Verification items for this drawing (mm, ordinates from the low corner). Round coordinates to 2 decimals unless told otherwise and drop trailing zeros. Write each loop counter-clockwise with the first axis right and the second up, starting at its lowest first coordinate (ties: lowest second). Pieces come first, ordered by that corner, then holes. Notation, with made-up numbers: (-36.75, 31) -> (2.25, 31) arc R28 ccw to (2.25, 61) -> close; hole circle Ø4 at (59.25, -31.75). An arc over 180 degrees is marked (long way). One line per item, written item: value.
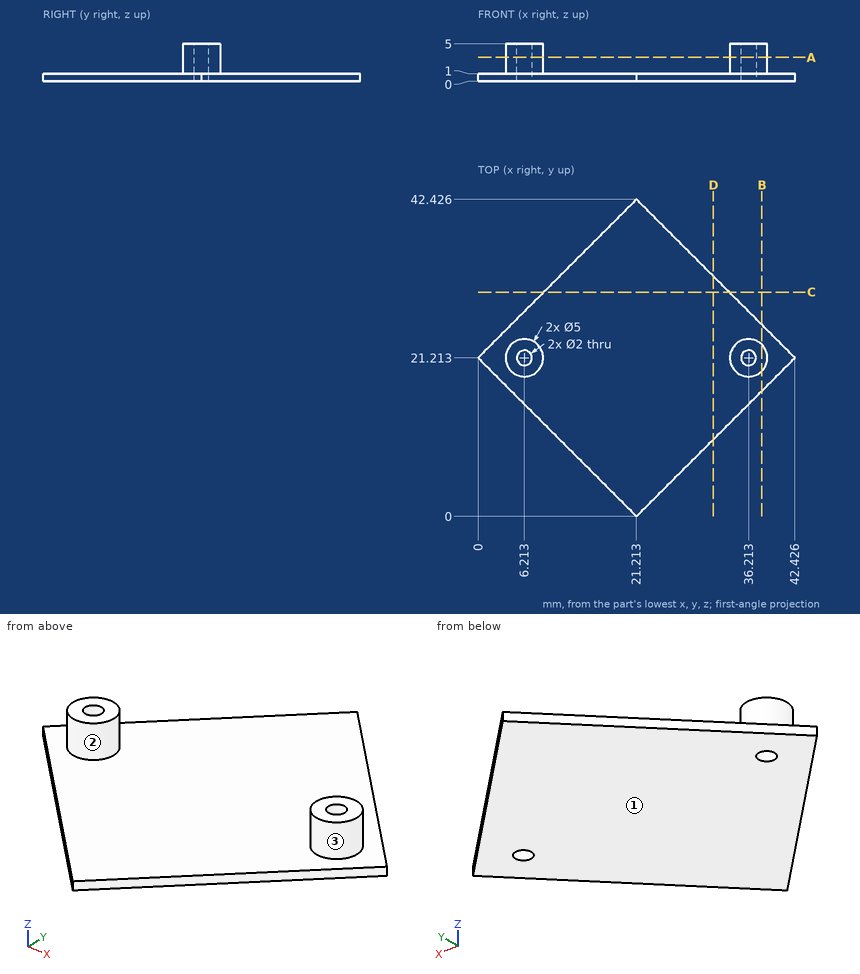
Item 1: Sectioned sample at A-A (z = 3.2). Enter the section's corners in (x, y), then the cut area to 3 significant figures.
Result set:
outline: circle Ø5 at (6.21, 21.21); circle Ø5 at (36.21, 21.21); hole circle Ø2 at (6.21, 21.21); hole circle Ø2 at (36.21, 21.21)
area: 33.0 mm^2
Item 2: Sectioned sample at B-B (x = 38). Enter the section's corners in (y, z) (1 decimal).
Result set:
outline: (16.8, 0) -> (25.6, 0) -> (25.6, 1) -> (23, 1) -> (23, 5) -> (19.5, 5) -> (19.5, 1) -> (16.8, 1) -> close
Item 3: Depth check by flat-ended pin: pin 1 (1 mm diameter, centred on y = 22, z = 3, fed in from -X); pin 2 (1.6 mm diameter, centred on x = 36.21, y = 21.21, fed in from +Z); pin 3 (10 mm diameter, centred on x = 35.5, y = 8, fed in from +Z); pin 4 (2.5 mm diameter, centred on x = 6.21, y = 21.21, fed in from +Z). Enter the tip coordinate at first touch or a pass-through.
Result set:
pin 1: x = 3.73
pin 2: through
pin 3: z = 1
pin 4: z = 5
Item 4: Sectioned sample at D-D (x = 31.5). Enter the section's corners in (y, z).
Result set:
outline: (10.29, 0) -> (32.14, 0) -> (32.14, 1) -> (10.29, 1) -> close
Item 5: Sectioned sample at C-C (y = 30). Enter the section's corners in (x, z).
Result set:
outline: (8.79, 0) -> (33.64, 0) -> (33.64, 1) -> (8.79, 1) -> close
Item 6: Release check for a two-part mould opening along X. For the marked faces 1, 2 and 3 record: pulls with the +X half, pulls with the -X half, needs draft (parallel to the pull), parting line crosses it, or undercut.
Result set:
face 1: needs draft
face 2: undercut
face 3: undercut
Item 7: Material ranges on line 1 along Z through (x, y) = (24.5, 30.5); line 2 along X through (y, z) = (20, 2); line 3 along Y through (x, z) = (31.5, 0.65) (1 decimal), recorded low to high.
Result set:
line 1: 0 to 1
line 2: 4.03 to 8.4, 34.03 to 38.4
line 3: 10.3 to 32.1
